from build123d import *

# Parameters (mm, degrees)
SKETCH_1_R               = 9.17
EXTRUDE_1_DEPTH          = 11
CUT_EXTRUDE_1_DEPTH      = 11
PATTERN_CIRCULAR_1_COUNT = 20
SKETCH_4_R               = 11
EXTRUDE_3_DEPTH          = 2
EXTRUDE_START            = 2
SKETCH_3_R               = 11
EXTRUDE_4_DEPTH          = 2
SKETCH_5_R               = 2.5
CUT_EXTRUDE_2_DEPTH      = 22


with BuildPart() as part:
    # 草图1 → 凸台-拉伸1 (new body)
    with BuildSketch(Plane(origin=(0, 0, 0), x_dir=(1, 0, 0), z_dir=(0, 1, 0))):
        with Locations(Location((0, 0, 0), (0, 0, 270))):
            Circle(SKETCH_1_R)
    extrude(amount=-EXTRUDE_1_DEPTH)

    # 草图2 → 切除-拉伸1 (cut)
    with BuildSketch(Plane(origin=(0, 0, 0), x_dir=(1, 0, 0), z_dir=(0, 1, 0))):
        with BuildLine():
            Line((-1.338469592, 9.071791397), (-1.301979145, 9.548134799))
            Line((-1.301979145, 9.548134799), (1.164461041, 9.508969944))
            Line((1.164461041, 9.508969944), (1.338469592, 9.071791397))
            ThreePointArc((1.338469592, 9.071791397), (1.164461041, 9.03324808), (1.06034373, 8.888596261))
            ThreePointArc((1.06034373, 8.888596261), (0, 8.072950826), (-1.06034373, 8.888596261))
            ThreePointArc((-1.06034373, 8.888596261), (-1.164461041, 9.03324808), (-1.338469592, 9.071791397))
        make_face()
    cut_extrude_1 = extrude(amount=-CUT_EXTRUDE_1_DEPTH, mode=Mode.SUBTRACT)

    # 阵列(圆周)1: 切除-拉伸1 ×20 about axis
    pattern_circular_1_axis = Axis((0, 0, 0), (0, 1, 0))
    for i in range(1, PATTERN_CIRCULAR_1_COUNT):
        add(cut_extrude_1.rotate(pattern_circular_1_axis, i * 360 / PATTERN_CIRCULAR_1_COUNT), mode=Mode.SUBTRACT)

    # 草图4 → 凸台-拉伸3 (add)
    with BuildSketch(Plane(origin=(0, 0, 0), x_dir=(1, 0, 0), z_dir=(0, 1, 0))):
        with Locations(Location((0, 0, 0), (0, 0, 270))):
            Circle(SKETCH_4_R)
    extrude(amount=EXTRUDE_3_DEPTH)

    # 草图3 → 凸台-拉伸4 (add)
    with BuildSketch(Plane.XZ.offset(11).offset(EXTRUDE_START)):
        with Locations(Location((0, 0, 0), (0, 0, 90))):
            Circle(SKETCH_3_R)
    extrude(amount=-EXTRUDE_4_DEPTH)

    # 草图5 → 切除-拉伸2 (cut)
    with BuildSketch(Plane(origin=(0, 2, 0), x_dir=(1, 0, 0), z_dir=(0, 1, 0))):
        with Locations(Location((0, 0, 0), (0, 0, 270))):
            Circle(SKETCH_5_R)
    extrude(amount=-CUT_EXTRUDE_2_DEPTH, mode=Mode.SUBTRACT)


solid = part.part
Could you check a few things on this model? Use its own coordinates, in mm. A direction names the side the tool comes from. Coordinates: 2 decimals unless noted, no trailing zeros. Order: outer loops, then holes, each group sorted by start corner. A loop starts at its lowest first (then second) coordinate and runs counter-clockwise, first axis right, second up. Notation, with made-up numbers: (62, 78.5) - (97, 78.5) arc R24 cw to (97, 105.5) - close; hole circle Ø6 at (68.25, -39). An arc over 180 degrees is marked (long way). Answer in a Markdown table with one row per item. Add a question column.
(1) If we section it at B-B, the plane x = 0: Please give me the cut outline in (y, z), then the cut area to 3 significant figures.
(2) I need wall thicknesses on L1, parallel to Y at x = 2.5, z = -8.25; L2, parallel to Z at x = 7.75, y = -7.5; L3, parallel to X at y = -1.5, z = 8. Which ranges of each line are inside material? Lowest first, please.
(3) Will these pins go through, and if not, where does the flat tip stop? pin 1 (4.5 mm diameter, centred on x = 0, z = 0, fed in from +Y); pin 2 (2 mm diameter, centred on y = -8, z = -4.5, fed in from +X); pin 3 (6 mm diameter, centred on y = -2.5, z = -1.5, fed in from -X); pin 4 (1 mm diameter, centred on x = -1.5, y = -5.5, fed in from -Z).
(4) If we section it at A-A, the plane z = 0: Please give me the cut outline in (x, y).
(5) If we mould it in two halves opening along X, with no side actions, what happens to faces 3 (the face through (-8.073, -5.423, -0.02)), 4 (the face through (-10.74, 0.99, -2.38)), 5 (the face through (-0.02, -5.423, 8.073))? For each: released by +X, released by -X, zero draft, split by the parting line, or undercut.
(6) If we section it at D-D, the plane x = -9.5: Please give me the cut outline in (y, z).
(7) On a 3-axis mill with a long thin cutter (end or side, diameter ignored), from which of +Z, -Z, +X, -X, +Y, -Y can I reach the whole of each face in a straight line? I mean faces 1 (the face through (4.76, -5.42, -6.52)), 2 (the face through (10.74, -12.01, -2.38)). Say none if no direction works.
(8) If we section it at C-C, the plane z = -9.5: Please give me the cut outline in (x, y).
Results are:
| question | item | result |
|---|---|---|
| 1 | outline | (-13, -11) - (-11, -11) - (-11, -8.07) - (0, -8.07) - (0, -11) - (2, -11) - (2, -2.5) - (-13, -2.5) - close; (-13, 2.5) - (2, 2.5) - (2, 11) - (0, 11) - (0, 8.07) - (-11, 8.07) - (-11, 11) - (-13, 11) - close |
| 1 | area | 191 mm2 |
| 2 | L1 | y = -13 to -11, 0 to 2 |
| 2 | L2 | z = -4.34 to -3.34, -2.32 to 2.32, 3.34 to 4.34 |
| 2 | L3 | x = -4.36 to -3.66, -2.01 to 2.01, 3.66 to 4.36 |
| 3 | pin 1 | passes through |
| 3 | pin 2 | stops at x = 8.24 |
| 3 | pin 3 | stops at x = -11 |
| 3 | pin 4 | stops at z = -9.07 |
| 4 | outline | (-11, -13) - (-2.5, -13) - (-2.5, 2) - (-11, 2) - (-11, 0) - (-8.07, 0) - (-8.07, -11) - (-11, -11) - close; (2.5, -13) - (11, -13) - (11, -11) - (8.07, -11) - (8.07, 0) - (11, 0) - (11, 2) - (2.5, 2) - close |
| 5 | face 3 | released by -X |
| 5 | face 4 | split by the parting line |
| 5 | face 5 | undercut |
| 6 | outline | (-13, -5.55) - (-11, -5.55) - (-11, 5.55) - (-13, 5.55) - close; (0, -5.55) - (2, -5.55) - (2, 5.55) - (0, 5.55) - close |
| 7 | face 1 | none |
| 7 | face 2 | +Y, -Y |
| 8 | outline | (-5.55, -13) - (5.55, -13) - (5.55, -11) - (-5.55, -11) - close; (-5.55, 0) - (5.55, 0) - (5.55, 2) - (-5.55, 2) - close |
